```python
from build123d import *

# Parameters (mm, degrees)
SKETCH_R      = 1.5
PAD_DEPTH     = 4
SKETCH001_R   = 3
SKETCH001_R_2 = 1.5
POCKET_DEPTH  = 1.5


with BuildPart() as part:
    # Sketch → Pad (new body)
    with BuildSketch(Plane.XY):
        with BuildLine():
            ThreePointArc((4.5, 27.2), (0, 31.7), (-4.5, 27.2))
            Line((-4.5, -27.2), (-4.5, 27.2))
            ThreePointArc((-4.5, -27.2), (0, -31.7), (4.5, -27.2))
            Line((4.5, 27.2), (4.5, -27.2))
        make_face()
        with Locations((0, 27.2)):
            Circle(SKETCH_R, mode=Mode.SUBTRACT)
        with Locations((0, -27.2)):
            Circle(SKETCH_R, mode=Mode.SUBTRACT)
    extrude(amount=PAD_DEPTH)

    # Sketch001 → Pocket (cut, symmetric)
    with BuildSketch(Plane.XY):
        with Locations((0, -27.2)):
            Circle(SKETCH001_R)
        with Locations((0, -27.2)):
            Circle(SKETCH001_R_2, mode=Mode.SUBTRACT)
        with Locations((0, 27.2)):
            Circle(SKETCH001_R)
        with Locations((0, 27.2)):
            Circle(SKETCH001_R_2, mode=Mode.SUBTRACT)
    extrude(amount=POCKET_DEPTH, both=True, mode=Mode.SUBTRACT)


solid = part.part
```
Work out the finished part from the listing and answer in its coordinate system (mm). A direction names the side the tool comes from. Round coordinates to 2 decimals unless told otherwise and drop trailing zeros. Loops run counter-clockwise (first coordinate to the right, second up) from the corner with the lowest first, then second, coordinate; pieces in that order, holes last.
(1) Find the intervals of material crossed by L1, parallel to Y at x = 0, z = 2.5; L2, parallel to Y at x = 0.25, z = 0.35; L3, parallel to Y at x = 3, z = 1.5, in increasing order.
Computed values:
L1: y = -31.7 to -28.7, -25.7 to 25.7, 28.7 to 31.7
L2: y = -31.69 to -30.19, -24.21 to 24.21, 30.19 to 31.69
L3: y = -30.55 to 30.55
(2) The mould has two halves that part along Y. Classify faces 1 (the cylindrical face through (0.806, -25.935, 2.732)), 2 (the cylindrical face through (-0.391, 30.174, 0.76)), 3 (the flat face through (0, 0, 4)), 4 (the cylindrical face through (0.1, 31.7, 2)): pulls with the +Y half, pulls with the -Y half, needs draft (parallel to the pull), parting line crosses it, or undercut.
Computed values:
face 1: undercut
face 2: undercut
face 3: needs draft
face 4: pulls with the +Y half
(3) The part is cut by section C-C, the plane x = 2.25. Give the vertices of the cut face in (y, z).
Computed values:
outline: (-31.1, 0) - (-29.18, 0) - (-29.18, 1.5) - (-25.22, 1.5) - (-25.22, 0) - (25.22, 0) - (25.22, 1.5) - (29.18, 1.5) - (29.18, 0) - (31.1, 0) - (31.1, 4) - (-31.1, 4) - close
(4) The part is cut by section A-A, the plane x = 0. Give the vertices of the cut face in (y, z), and give its area (3 significant figures).
Computed values:
outline: (-31.7, 0) - (-30.2, 0) - (-30.2, 1.5) - (-28.7, 1.5) - (-28.7, 4) - (-31.7, 4) - close; (-25.7, 1.5) - (-24.2, 1.5) - (-24.2, 0) - (24.2, 0) - (24.2, 1.5) - (25.7, 1.5) - (25.7, 4) - (-25.7, 4) - close; (28.7, 1.5) - (30.2, 1.5) - (30.2, 0) - (31.7, 0) - (31.7, 4) - (28.7, 4) - close
area: 221 mm2
(5) For faces 5 (the flat face through (4.5, 0, 2)), 6 (the flat face through (1, 29, 1.5)), determine the directions among +Z, -Z, +X, -X, +Y, -Y from which every point of the face is accessible in a straight line to the end or side of a thin tool.
Computed values:
face 5: +Z, -Z, +X, +Y, -Y
face 6: -Z
(6) The part is cut by section B-B, the plane z = 0.7. Give the vertices of the cut face in (x, y), and give its area (3 significant figures).
Computed values:
outline: (-4.5, -27.2) arc R4.5 ccw to (4.5, -27.2) - (4.5, 27.2) arc R4.5 ccw to (-4.5, 27.2) - close; hole circle Ø6 at (0, -27.2); hole circle Ø6 at (0, 27.2)
area: 497 mm2
(7) This flat-tipped pin is pushed along its axis until it touches: P1, Ø1.8, axis at x = 0, y = -26.5, coming from the -Z side. Where does it stop, or does it pass through?
Computed values:
P1: stops at z = 1.5
